Part model, mm, in its own coordinate system. Face numbers are marked on the shaded views. A direction names the side the tool comes from. Round coordinates to 2 decimals unless told otherwise and drop trailing zeros. Write each loop counter-clockwise with the first axis right and the second up, starting at its lowest first coordinate (ties: lowest second). Pieces come first, ordered by that corner, then holes. Notation, with made-up numbers: M -16.75,-23.5 L 42.25,-23.5 A12 ccw 42.25,-13.5 Z; hole C 1,74 d1. An arc over 180 degrees is marked long. One line per question, with ' | ' between items. Start each with the question number.
1) Saw through at A-A (z = -12). List the corners of the cut face in (x, y), plus the area to 3 significant figures.
2) Wall check: probe 1 along X at (y, z) = (0.5, 14.5); probe 2 along X at (y, z) = (13.3, -12); probe 3 along Y at (x, z) = (11.5, 6). Give the ranges that are in metal, low to high. Write a range as [from, to].
3) Saw through at D-D (y = 1.5). List the corners of the cut face in (x, z).
4) Saw through at B-B (x = 2.5). List the corners of the cut face in (y, z), plus the area to 3 significant figures.
5) Saw through at C-C (z = 14). List the corners of the cut face in (x, y), plus the area to 3 significant figures.
6) Tool access for the marked faces 1, 2 and 3: list every direction of +Z, -Z, +X, -X, +Y, -Y with a clear straight run to the whole face (end or side of a thin tool).
7) Mould opens along Y. For the marked faces 4, 5 and 6 say: pulls with the +Y half, pulls with the -Y half, needs draft (parallel to the pull), parting line crosses it, or undercut.
8) Drop flat-ended pins along their axis: pin 1 Ø10 at (x, z) = (2, -14.5) entering from -Y; pin 2 Ø4 at (x, z) = (6.5, 13.5) entering from +Y; pin 3 Ø6.5 at (x, y) = (7.5, 0.5) entering from -Z. Give the stop position or say it passes through.
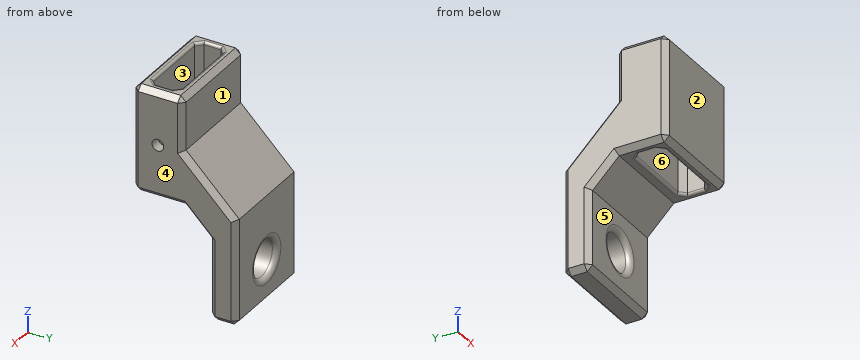
```python
from build123d import *

# Parameters (mm, degrees)
ESBO_O2_W                = 19.4
ESBO_O2_H                = 9.4
RESSALTO_EXTRUS_O1_DEPTH = 20
RESSALTO_EXTRUS_O2_DEPTH = 19.4
CHANFRO2_SIZE            = 1
ESBO_O5_R                = 3.5
CORTE_EXTRUS_O1_DEPTH    = 20
FILETE1_R                = 1
FILETE2_R                = 0.5
ESBO_O6_R                = 1.1
CORTE_EXTRUS_O2_DEPTH    = 10


with BuildPart() as part:
    # Esboço2 → Ressalto-extrusão1 (new body)
    with BuildSketch(Plane.XY):
        with Locations((7.5, 1.5)):
            Rectangle(ESBO_O2_W, ESBO_O2_H)
        Polygon((15.2, 3.082842712), (14.082842712, 4.2), (0.917157288, 4.2), (-0.2, 3.082842712), (-0.2, -0.082842712), (0.917157288, -1.2), (14.082842712, -1.2), (15.2, -0.082842712), align=None, mode=Mode.SUBTRACT)
    extrude(amount=RESSALTO_EXTRUS_O1_DEPTH)

    # Esboço4 → Ressalto-extrusão2 (add)
    with BuildSketch(Plane(origin=(-2.2, 0, 0), x_dir=(0, 0, -1), z_dir=(1, 0, 0))):
        Polygon((0, 16.2), (-10, 6.2), (0, 6.2), (5, 11.2), (20, 11.2), (20, 16.2), align=None)
    extrude(amount=RESSALTO_EXTRUS_O2_DEPTH)

    # Chanfro2
    chanfro2_edges = [part.edges().sort_by_distance(p)[0] for p in [
        (17.2, 1.5, 20),
        (7.5, 6.2, 20),
        (17.2, 11.2, 5),
        (-2.2, 11.2, 5),
        (17.2, 8.7, -2.5),
        (-2.2, 8.7, -2.5),
        (17.2, 11.2, -12.5),
        (-2.2, 11.2, -12.5),
        (17.2, 13.7, -20),
        (7.5, 11.2, -20),
        (-2.2, 13.7, -20),
        (7.5, 16.2, -20),
        (-2.2, 16.2, -10),
        (17.2, 16.2, -10),
        (-2.2, 1.5, 20),
        (17.2, 1.5, 0),
        (7.5, -3.2, 0),
        (-2.2, 1.5, 0),
        (-2.2, 6.2, 15),
        (17.2, 6.2, 15),
        (17.2, -3.2, 10),
        (-2.2, -3.2, 10),
        (7.5, -3.2, 20),
    ]]
    chamfer(chanfro2_edges, length=CHANFRO2_SIZE)

    # Esboço5 → Corte-extrusão1 (cut)
    with BuildSketch(Plane.XZ.offset(-11.2)):
        with Locations(Location((7.5, -12, 0), (0, 0, 270))):
            Circle(ESBO_O5_R)
    extrude(amount=-CORTE_EXTRUS_O1_DEPTH, mode=Mode.SUBTRACT)

    # Filete1
    filete1_edges = [part.edges().sort_by_distance(p)[0] for p in [
        (7.5, 16.2, -8.5),
        (7.5, 11.2, -8.5),
    ]]
    fillet(filete1_edges, radius=FILETE1_R)

    # Filete2
    filete2_edges = [part.edges().sort_by_distance(p)[0] for p in [
        (15.2, 1.5, 0),
        (14.641421356, 3.641421356, 0),
        (7.5, 4.2, 0),
        (0.358578644, 3.641421356, 0),
        (-0.2, 1.5, 0),
        (0.358578644, -0.641421356, 0),
        (7.5, -1.2, 0),
        (14.641421356, -0.641421356, 0),
        (15.2, 1.5, 20),
        (14.641421356, 3.641421356, 20),
        (7.5, 4.2, 20),
        (0.358578644, 3.641421356, 20),
        (-0.2, 1.5, 20),
        (0.358578644, -0.641421356, 20),
        (7.5, -1.2, 20),
        (14.641421356, -0.641421356, 20),
    ]]
    fillet(filete2_edges, radius=FILETE2_R)

    # Esboço6 → Corte-extrusão2 (cut)
    with BuildSketch(Plane(origin=(17.2, 0, 0), x_dir=(0, 0, -1), z_dir=(1, 0, 0))):
        with Locations((-10, 1.5)):
            Circle(ESBO_O6_R)
    extrude(amount=-CORTE_EXTRUS_O2_DEPTH, mode=Mode.SUBTRACT)


solid = part.part
```
Answer key:
1) outline: M -2.2,12.2 L -1.2,11.2 L 3,11.2 A1 ccw 4,12.2 L 4,15.2 A1 ccw 3,16.2 L -1.2,16.2 L -2.2,15.2 Z; M 11,12.2 A1 ccw 12,11.2 L 16.2,11.2 L 17.2,12.2 L 17.2,15.2 L 16.2,16.2 L 12,16.2 A1 ccw 11,15.2 Z | area: 59.1 mm2
2) probe 1: x = [-2.2, -0.2], [15.2, 17.2] | probe 2: x = [-2.2, 4], [11, 17.2] | probe 3: y = [-3.2, -1.2], [4.2, 10.2]
3) outline: M -2.2,1 L -1.2,0 L -0.7,0 A0.5 ccw -0.2,0.5 L -0.2,19.5 A0.5 ccw -0.7,20 L -1.2,20 L -2.2,19 Z; M 15.2,0.5 A0.5 ccw 15.7,0 L 16.2,0 L 17.2,1 L 17.2,8.9 L 15.2,8.9 Z; M 15.2,11.1 L 17.2,11.1 L 17.2,19 L 16.2,20 L 15.7,20 A0.5 ccw 15.2,19.5 Z
4) outline: M -3.2,1 L -2.2,0 L -1.7,0 A0.5 ccw -1.2,0.5 L -1.2,19.5 A0.5 ccw -1.7,20 L -2.2,20 L -3.2,19 Z; M 4.2,0.5 A0.5 ccw 4.7,0 L 6.2,0 L 11.2,-5 L 11.2,-19 L 12.2,-20 L 15.2,-20 L 16.2,-19 L 16.2,0 L 6.2,10 L 6.2,19 L 5.2,20 L 4.7,20 A0.5 ccw 4.2,19.5 Z | area: 240 mm2
5) outline: M -2.2,-2.2 L -1.2,-3.2 L 16.2,-3.2 L 17.2,-2.2 L 17.2,5.2 L 16.2,6.2 L -1.2,6.2 L -2.2,5.2 Z; hole M -0.2,-0.08 L 0.92,-1.2 L 14.08,-1.2 L 15.2,-0.08 L 15.2,3.08 L 14.08,4.2 L 0.92,4.2 L -0.2,3.08 Z | area: 99.7 mm2
6) face 1: +Z, +X, -X, +Y | face 2: +Z, -Z, +X, -X, -Y | face 3: +Z, -Z
7) face 4: needs draft | face 5: pulls with the -Y half | face 6: undercut
8) pin 1: stops at y = 11.2 | pin 2: stops at y = 6.2 | pin 3: stops at z = 0
